from build123d import *

# Parameters (mm, degrees)
F0_W     = 96.166272
F0_H     = 101.375278
F1_DEPTH = 40
F3_DEPTH = 40
F4_R     = 5
F5_DEPTH = 40.001


with BuildPart() as f1:
    # F0 (on Front) → F1 (new body)
    with BuildSketch(Plane.XZ):
        with Locations((-7.412447, 4.371865)):
            Rectangle(F0_W, F0_H)
    extrude(amount=F1_DEPTH)

    # F2 (on face) → F3 (join)
    with BuildSketch(Plane.XZ.offset(40)):
        Polygon((-93.307483, 11.53077), (-55.495583, -26.281131), (-55.495583, 11.53077), align=None)
    extrude(amount=-F3_DEPTH)

    # F4 (on face) → F5 (cut, through all)
    with BuildSketch(Plane(origin=(0, 0, 0), x_dir=(-1, 0, 0), z_dir=(0, 1, 0))):
        with Locations((38.787491, -27.369825)):
            Circle(F4_R)
        with Locations((-25.670689, -31.315774)):
            Circle(F4_R)
        with Locations((-25.670689, 40.059504)):
            Circle(F4_R)
        with Locations((40.495583, 39.617617)):
            Circle(F4_R)
    extrude(amount=-F5_DEPTH, mode=Mode.SUBTRACT)


solid = f1.part
Work out the finished part from the listing and answer in its coordinate system (mm). A direction names the side the tool comes from. Coordinates: 2 decimals unless noted, no trailing zeros. Write each loop counter-clockwise with the first axis right and the second up, starting at its lowest first coordinate (ties: lowest second). Pieces come first, ordered by that corner, then holes.
1. Flat-ended cylindrical pins translate along their axes: pin 1 (13 mm diameter, centred on x = 25.67, z = 40.06, fed in from +Y); pin 2 (6 mm diameter, centred on y = -19.5, z = -24.5, fed in from -X); pin 3 (19 mm diameter, centred on x = -71, y = -23, fed in from +Z); pin 4 (1 mm diameter, centred on y = -11.5, z = -17.5, fed in from -X). Find the tip coordinate at first contact, or state that the pin passes through.
Results list:
pin 1: stops at y = 0
pin 2: stops at x = -60.28
pin 3: stops at z = 11.53
pin 4: stops at x = -64.78
2. For a pull along Z with two mould halves and no side action, classify faces 1 (the flat face through (-55.496, -20, -36)), 2 (the cylindrical face through (29.356, -19.72, 43.439)), 3 (the flat face through (-74, -20, 11.531)) as +Z half, -Z half, draft (parallel to the pull), parting line (faces both ways), or undercut.
Results list:
face 1: draft
face 2: undercut
face 3: +Z half
3. Consider line 1 along X through (y, z) = (-15.5, 36.5); line 2 along X through (y, z) = (-32, -31.5); line 3 along X through (y, z) = (-33.5, 31). Determine where each line is inside the solid, lowest interval first.
Results list:
line 1: x = -55.5 to -44.4, -36.59 to 22.16, 29.18 to 40.67
line 2: x = -55.5 to -41.61, -35.97 to 20.67, 30.67 to 40.67
line 3: x = -55.5 to 40.67
4. For faces 4 (the flat face through (-55.496, -20, 33)), 5 (the flat face through (40.671, -20, 4)), determine the directions among +Z, -Z, +X, -X, +Y, -Y from which every point of the face is accessible in a straight line to the end or side of a thin tool.
Results list:
face 4: +Z, -X, +Y, -Y
face 5: +Z, -Z, +X, +Y, -Y
5. The part is cut by section C-C, the plane z = 47.5. Write down the section's boundary in (x, y).
Results list:
outline: (-55.5, -40) - (40.67, -40) - (40.67, 0) - (-55.5, 0) - close
6. The part is cut by section A-A, the plane x = -39.5. Write down the section's boundary in (y, z), and give its area (3 significant figures).
Results list:
outline: (-40, -46.32) - (0, -46.32) - (0, -32.32) - (-40, -32.32) - close; (-40, -22.42) - (0, -22.42) - (0, 34.72) - (-40, 34.72) - close; (-40, 44.52) - (0, 44.52) - (0, 55.06) - (-40, 55.06) - close
area: 3,270 mm2
7. The part is cut by section D-D, the plane x = -81.5. Write down the section's boundary in (y, z).
Results list:
outline: (-40, -0.28) - (0, -0.28) - (0, 11.53) - (-40, 11.53) - close
8. The part is cut by section B-B, the plane y = -13.5. Write down the section's boundary in (x, z), and give its area (3 significant figures).
Results list:
outline: (-93.31, 11.53) - (-55.5, -26.28) - (-55.5, -46.32) - (40.67, -46.32) - (40.67, 55.06) - (-55.5, 55.06) - (-55.5, 11.53) - close; hole circle Ø10 at (-40.5, 39.62); hole circle Ø10 at (-38.79, -27.37); hole circle Ø10 at (25.67, -31.32); hole circle Ø10 at (25.67, 40.06)
area: 10,100 mm2
